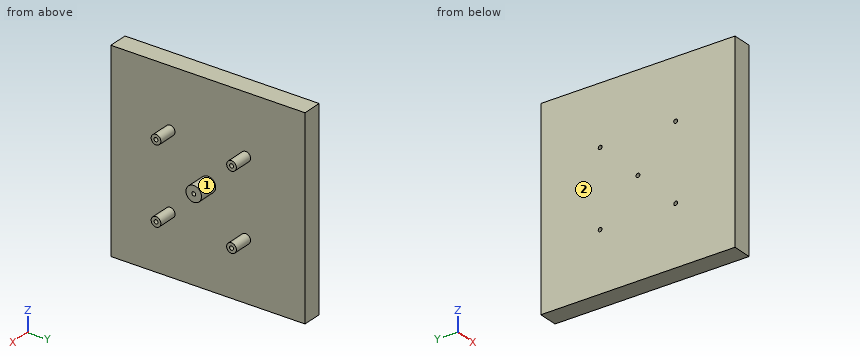
from build123d import *

# Parameters (mm, degrees)
SKETCH1_W           = 100
SKETCH1_H           = 100
SKETCH1_R           = 1
BOSS_EXTRUDE2_DEPTH = 10
SKETCH2_R           = 4
SKETCH2_R_2         = 1
SKETCH2_R_3         = 2.5
BOSS_EXTRUDE3_DEPTH = 10


with BuildPart() as part:
    # Sketch1 → Boss-Extrude2 (new body)
    with BuildSketch(Plane(origin=(0, 0, 0), x_dir=(0, 0, -1), z_dir=(1, 0, 0))):
        Rectangle(SKETCH1_W, SKETCH1_H)
        with Locations((19.445436483, 19.445436483)):
            Circle(SKETCH1_R, mode=Mode.SUBTRACT)
        with Locations((19.445436483, -19.445436483)):
            Circle(SKETCH1_R, mode=Mode.SUBTRACT)
        with Locations((-19.445436483, -19.445436483)):
            Circle(SKETCH1_R, mode=Mode.SUBTRACT)
        with Locations((-19.445436483, 19.445436483)):
            Circle(SKETCH1_R, mode=Mode.SUBTRACT)
        Circle(SKETCH1_R, mode=Mode.SUBTRACT)
    extrude(amount=BOSS_EXTRUDE2_DEPTH)

    # Sketch2 → Boss-Extrude3 (add)
    # profile 1 of 5: a face of its own
    with BuildSketch(Plane(origin=(10, 0, 0), x_dir=(0, 0, -1), z_dir=(1, 0, 0))):
        Circle(SKETCH2_R)
        Circle(SKETCH2_R_2, mode=Mode.SUBTRACT)
    # profile 2 of 5: a face of its own
    with BuildSketch(Plane(origin=(10, 0, 0), x_dir=(0, 0, -1), z_dir=(1, 0, 0))):
        with Locations((19.445436483, 19.445436483)):
            Circle(SKETCH2_R_3)
        with Locations((19.445436483, 19.445436483)):
            Circle(SKETCH2_R_2, mode=Mode.SUBTRACT)
    # profile 3 of 5: a face of its own
    with BuildSketch(Plane(origin=(10, 0, 0), x_dir=(0, 0, -1), z_dir=(1, 0, 0))):
        with Locations((19.445436483, -19.445436483)):
            Circle(SKETCH2_R_3)
        with Locations((19.445436483, -19.445436483)):
            Circle(SKETCH2_R_2, mode=Mode.SUBTRACT)
    # profile 4 of 5: a face of its own
    with BuildSketch(Plane(origin=(10, 0, 0), x_dir=(0, 0, -1), z_dir=(1, 0, 0))):
        with Locations((-19.445436483, -19.445436483)):
            Circle(SKETCH2_R_3)
        with Locations((-19.445436483, -19.445436483)):
            Circle(SKETCH2_R_2, mode=Mode.SUBTRACT)
    # profile 5 of 5: a face of its own
    with BuildSketch(Plane(origin=(10, 0, 0), x_dir=(0, 0, -1), z_dir=(1, 0, 0))):
        with Locations((-19.445436483, 19.445436483)):
            Circle(SKETCH2_R_3)
        with Locations((-19.445436483, 19.445436483)):
            Circle(SKETCH2_R_2, mode=Mode.SUBTRACT)
    extrude(amount=BOSS_EXTRUDE3_DEPTH)


solid = part.part
The model under review builds one solid part; all positions refer to its coordinate system, in mm. Face numbers are marked on the shaded views. A direction names the side the tool comes from. Give positions to 0.01 mm unless a question says otherwise; leave off trailing zeros. Write each loop counter-clockwise with the first axis right and the second up, starting at its lowest first coordinate (ties: lowest second). Pieces come first, ordered by that corner, then holes.
1. Tool access review of the marked faces 1 and 2: name each direction out of +Z, -Z, +X, -X, +Y, -Y from which nothing blocks a thin tool from reaching the whole face with its end or side.
2. Wall thickness on L1, parallel to Y at x = 10.75, z = -20; L2, parallel to X at y = 17.5, z = 40.5; L3, parallel to Y at x = 17.5, z = 3.5: over which ranges is each line inside the solid? List them lowest first.
3. Add section A-A, the plane x = 13.5. Count the separate pieces of the cut face and the enclosed holes in it, plus the area to 3 significant figures.
4. For P1, Ø2, axis at x = 17.5, y = 6, coming from the -Z side; P2, Ø1, axis at y = 10, z = 6.5, coming from the +X side, all flat-tipped, find the tip position at first contact; note any pin that passes through.
5. Add section B-B, the plane y = -31. Write out the cut boundary in (x, z), plus the area to 3 significant figures.
Worked answers:
1. face 1: +X
1. face 2: +Z, -Z, -X, +Y, -Y
2. L1: y = -21.88 to -20.28, -18.61 to -17.01, 17.01 to 18.61, 20.28 to 21.88
2. L2: x = 0 to 10
2. L3: y = -1.94 to 1.94
3. separate pieces: 5
3. enclosed holes: 5
3. area: 113 mm2
4. P1: passes through
4. P2: stops at x = 10
5. outline: (0, -50) - (10, -50) - (10, 50) - (0, 50) - close
5. area: 1,000 mm2
